from build123d import *

# Parameters (mm, degrees)
BOSS_EXTRUDE1_DEPTH = 38
SKETCH2_R           = 6.5
CUT_EXTRUDE1_DEPTH  = 58
FILLET1_R           = 1.25


with BuildPart() as part:
    # Sketch1 → Boss-Extrude1 (new body)
    with BuildSketch(Plane.XY):
        with BuildLine():
            Line((-9.5, 0), (9.5, 0))
            Line((9.5, 0), (9.5, 38))
            Line((9.5, 38), (8.25, 38))
            ThreePointArc((8.25, 38), (7.366116524, 37.633883476), (7, 36.75))
            Line((7, 36.75), (7, 2.5))
            Line((7, 2.5), (-7, 2.5))
            Line((-7, 2.5), (-7, 36.75))
            ThreePointArc((-7, 36.75), (-7.366116524, 37.633883476), (-8.25, 38))
            Line((-8.25, 38), (-9.5, 38))
            Line((-9.5, 38), (-9.5, 0))
        make_face()
    extrude(amount=BOSS_EXTRUDE1_DEPTH)

    # Sketch2 → Cut-Extrude1 (cut, through all)
    with BuildSketch(Plane(origin=(9.5, 0, 0), x_dir=(0, 0, -1), z_dir=(1, 0, 0))):
        with Locations((-19, 25)):
            Circle(SKETCH2_R)
    extrude(amount=-CUT_EXTRUDE1_DEPTH, mode=Mode.SUBTRACT)

    # Fillet1
    fillet1_edges = [part.edges().sort_by_distance(p)[0] for p in [
        (7.366116524, 37.633883476, 0),
        (-7.366116524, 37.633883476, 0),
        (9.5, 19, 38),
        (0, 0, 38),
        (-9.5, 19, 38),
        (-7.366116524, 37.633883476, 38),
        (-7, 19.625, 38),
        (0, 2.5, 38),
        (7, 19.625, 38),
        (7.366116524, 37.633883476, 38),
        (7, 19.625, 0),
        (9.5, 19, 0),
        (0, 0, 0),
        (0, 2.5, 0),
        (-7, 19.625, 0),
        (-9.5, 19, 0),
        (-9.5, 38, 19),
        (9.5, 38, 19),
    ]]
    fillet(fillet1_edges, radius=FILLET1_R - 0.0001)  # a hair under: the kernel refuses the full size


solid = part.part
Geometry check sheet. Reference: the model listing, model coordinates, mm. A direction names the side the tool comes from. Give positions to 0.01 mm unless a question says otherwise; leave off trailing zeros. Answer as a JSON object with one key per item and string values. Group by question number.
Item 1: Access from +Z, -Z, +X, -X, +Y, -Y to the whole of each face (thin tool, end or side, straight path). Record for faces 5 (the flat face through (-7, 16, 19)), 6 (the flat face through (9.5, 18, 19)).
Item 2: Mould release check, pull along X, two halves, no side actions. Record for faces 1 (the cylindrical face through (-0.115, 2.124, 37.644)), 2 (the cylindrical face through (9.144, 18.632, 0.376)), 3 (the cylindrical face through (7.376, 18.752, 37.644)), 4 (the cylindrical face through (-9.144, 37.624, 19.249)): pulls with the +X half, pulls with the -X half, needs draft (parallel to the pull), parting line crosses it, or undercut.
Item 3: Sectioned sample at A-A on z = 19. Give the number of separate pieces and of enclosed holes in the cut face, plus the area to 3 significant figures.
Item 4: Gauge pin test, flat ends, axial feed: pin 1 (8 mm diameter, centred on x = -3.5, z = 10, fed in from +Y); pin 2 (6 mm diameter, centred on x = -3.5, z = 13, fed in from +Y). Record the tip position at first contact, or that the pin passes through.
Item 5: Material ranges on L1, parallel to X at y = 28, z = 5.5; L2, parallel to Y at x = 8.25, z = 19; L3, parallel to Y at x = -1.5, z = 20.5, recorded low to high.
Findings below:
{
 "1": {"face 5": "+Z, -Z, +Y", "face 6": "+Z, -Z, +X, +Y, -Y"},
 "2": {"face 1": "undercut", "face 2": "pulls with the +X half", "face 3": "undercut", "face 4": "pulls with the -X half"},
 "3": {"separate pieces": "3", "enclosed holes": "0", "area": "159 mm2"},
 "4": {"pin 1": "y = 37.75", "pin 2": "y = 2.5"},
 "5": {"L1": "-9.5 to -7, 7 to 9.5", "L2": "0 to 18.5, 31.5 to 38", "L3": "0 to 2.5"}
}
